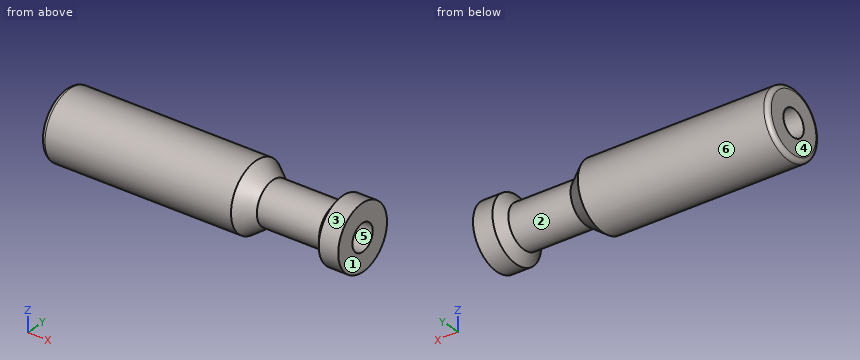
```python
from build123d import *

# Parameters (mm, degrees)
SKETCH4_R          = 7.9375
CUT_EXTRUDE1_DEPTH = 190.5
FILLET1_R          = 2.54


with BuildPart() as part:
    # Sketch1 → Revolve1 (revolve)
    with BuildSketch(Plane.XY):
        Polygon((107.503032851, -34.960925594), (117.452183803, -42.243603137), (154.81866926, -42.243603137), (159.466804827, -35.893603137), (171.145497316, -35.893603137), (171.145497316, -54.943603137), (-6.654502684, -54.943603137), (-6.654502684, -34.960925594), align=None)
    revolve(axis=Axis((171.145497316, -54.943603137, 0), (-1, 0, 0)))

    # Sketch4 → Cut-Extrude1 (cut)
    with BuildSketch(Plane(origin=(171.145497316, 0, 0), x_dir=(0, 0, -1), z_dir=(1, 0, 0))):
        with Locations(Location((0, -54.943603137, 0), (0, 0, 90))):
            Circle(SKETCH4_R)
    extrude(amount=-CUT_EXTRUDE1_DEPTH, mode=Mode.SUBTRACT)

    # Fillet1
    fillet1_edges = [part.edges().sort_by_distance(p)[0] for p in [
        (-6.654502684, -74.926280681, 0),
    ]]
    fillet(fillet1_edges, radius=FILLET1_R)


solid = part.part
```
CAD build for the part. Positions are in the model's coordinates, mm. Face numbers are marked on the shaded views. A direction names the side the tool comes from. Round coordinates to 2 decimals unless told otherwise and drop trailing zeros. Loops run counter-clockwise (first coordinate to the right, second up) from the corner with the lowest first, then second, coordinate; pieces in that order, holes last. Notation, with made-up numbers: (79, 69.5) - (119, 69.5) arc R9 ccw to (119, 77.5) - close; hole circle Ø10 at (54, -13.5). An arc over 180 degrees is marked (long way). Return JSON: item names as keys, results as strings. Group by question number.
Q1. Band-saw the part on B-B on x = 65. Give the cut face in (y, z) (1 decimal), plus the area to 3 significant figures.
Q2. Flat gauge pins, fed straight in: pin 1 Ø1 at (x, y) = (131.5, -50) entering from +Z; pin 2 Ø3 at (x, z) = (96, -13) entering from +Y; pin 3 Ø9.5 at (y, z) = (-54.94, 0) entering from +X; pin 4 Ø1.5 at (x, z) = (130, 1) entering from +Y. Where does each tip first touch, or does it go through?
Q3. Tool access for the marked faces 1, 2 and 3: list every direction of +Z, -Z, +X, -X, +Y, -Y with a clear straight run to the whole face (end or side of a thin tool).
Q4. Two-plate mould, pull along Y, no slides. Class the marked faces 4, 5 and 6: +Y half, -Y half, draft (parallel to the pull), parting line (faces both ways), or undercut.
Q5. Band-saw the part on C-C on x = 122.5. Give the cut face in (y, z) (1 decimal).
Q6. Drill centre lines: line 1 along Z through (x, y) = (11.5, -59); line 2 along X through (y, z) = (-48, -17); line 3 along X through (y, z) = (-60, 18). Where is each one in solid material? Low to high. Write a range as [from, to].
Q7. Band-saw the part on A-A on z = 0. Give the cut face in (x, y).
Solutions:
{
 "1": {"outline": "circle Ø40 at (-54.9, 0); hole circle Ø15.9 at (-54.9, 0)", "area": "1,060 mm^2"},
 "2": {"pin 1": "stops at z = 11.9", "pin 2": "stops at y = -38.6", "pin 3": "passes through", "pin 4": "stops at y = -42.25"},
 "3": {"face 1": "+Z, -Z, +X, +Y, -Y", "face 2": "none", "face 3": "+X"},
 "4": {"face 4": "draft", "face 5": "undercut", "face 6": "parting line"},
 "5": {"outline": "circle Ø25.4 at (-54.9, 0); hole circle Ø15.9 at (-54.9, 0)"},
 "6": {"line 1": "z = [-19.57, -6.82], [6.82, 19.57]", "line 2": "x = [-6.48, 109.72], [158.96, 171.15]", "line 3": "x = [-6.32, 109.26], [159.21, 171.15]"},
 "7": {"outline": "(-6.65, -72.39) arc R2.54 ccw to (-4.11, -74.93) - (107.5, -74.93) - (117.45, -67.64) - (154.82, -67.64) - (159.47, -73.99) - (171.15, -73.99) - (171.15, -62.88) - (-6.65, -62.88) - close; (-6.65, -47.01) - (171.15, -47.01) - (171.15, -35.89) - (159.47, -35.89) - (154.82, -42.24) - (117.45, -42.24) - (107.5, -34.96) - (-4.11, -34.96) arc R2.54 ccw to (-6.65, -37.5) - close"}
}
